Check sheet for the modelled part. Datum: model origin and axes. Units: mm. A direction names the side the tool comes from. Coordinates: 2 decimals unless noted, no trailing zeros. Loops run counter-clockwise (first coordinate to the right, second up) from the corner with the lowest first, then second, coordinate; pieces in that order, holes last. Notation, with made-up numbers: (-13, 32) - (22, 32) arc R35 ccw to (22, 65) - close; hole circle Ø1 at (83, 70.25). An arc over 180 degrees is marked (long way). Use a Markdown table: item, result. Add a question column.
1) Draft check along Y on faces 4 (the cylindrical face through (-3.78, -2.9, 21.41)), 5 (the flat face through (8, -8, 17.661)), 6 (the cylindrical face through (-0.448, 3.415, -33.518)). Enter one of: pulls with the +Y half, pulls with the -Y half, needs draft (parallel to the pull), parting line crosses it, or undercut.
2) Go/stop test with flat-tipped pins: P1, Ø3, axis at x = 0, y = 0, coming from the -Z side; P2, Ø3, axis at x = 1, y = -1, coming from the +Z side; P3, Ø8.5, axis at x = 0, y = 0, coming from the -Z side; P4, Ø8, axis at x = 22.5, y = -12, coming from the +Z side. Record where each tip stops, or that it passes through.
3) Tool access check on faces 1 (the cylindrical face through (25.034, 7.884, -11.992)), 2 (the flat face through (4, -4, 26.106)), 3 (the cylindrical face through (8.12, -3.37, 21.94)). Record the directions out of +Z, -Z, +X, -X, +Y, -Y that give a thin tool (end or side, any length) a straight path to the whole face; none if there is none.
4) Sectioned sample at A-A, the plane x = 24.5. Enter the section's corners in (y, z).
5) Sectioned sample at C-C, the plane z = -3. Enter the section's corners in (x, y), then the cut area to 3 significant figures.
6) Thickness scan on line 1 (Y direction, x = 0, z = 21); line 2 (Y direction, x = 0, z = -23); line 3 (Z direction, x = 28.5, y = 13.5). Record the ranges inside material, lowest first.
7) Sectioned sample at D-D, the plane z = -31.5. Enter the section's corners in (x, y) (1 decimal), then the cut area to 3 significant figures.
from build123d import *

# Parameters (mm, degrees)
F2_R     = 4.7625
F3_DEPTH = 9.525
F4_R     = 1.5875
F5_DEPTH = 22.225


with BuildPart() as f1:
    # F0 (on Front) → F1 (revolve)
    with BuildSketch(Plane.XZ):
        Polygon((8.793218, 26.10616), (0, 26.10616), (0, -37.513819), (3.444635, -37.513819), (3.444635, -29.631697), (7.104192, -29.631697), (7.104192, -21.186566), (16.393835, -21.186566), (16.393835, -15.274976), (26.246486, -15.274976), (26.246486, -8.800376), (33.565599, -8.800376), (33.565599, -4.296307), (36.099136, -4.296307), (36.099136, 17.661031), (8.793218, 17.661031), align=None)
    revolve(axis=Axis((0, 0, -5.703829), (0, 0, 1)))

    # F2 (on face) → F3 (cut)
    with BuildSketch(Plane.XY.offset(26.10616)):
        Circle(F2_R)
    extrude(amount=-F3_DEPTH, mode=Mode.SUBTRACT)

    # F4 (on face) → F5 (cut)
    with BuildSketch(Plane(origin=(0, 0, -37.513819), x_dir=(1, 0, 0), z_dir=(0, 0, -1))):
        Circle(F4_R)
    extrude(amount=-F5_DEPTH, mode=Mode.SUBTRACT)


solid = f1.part
Solved:
| question | item | result |
|---|---|---|
| 1 | face 4 | undercut |
| 1 | face 5 | needs draft |
| 1 | face 6 | parting line crosses it |
| 2 | P1 | stops at z = -15.29 |
| 2 | P2 | stops at z = 16.58 |
| 2 | P3 | stops at z = -37.51 |
| 2 | P4 | stops at z = 17.66 |
| 3 | face 1 | -Z |
| 3 | face 2 | +Z, +X, -X, +Y, -Y |
| 3 | face 3 | +Z |
| 4 | outline | (-26.51, -4.3) - (-22.94, -4.3) - (-22.94, -8.8) - (-9.41, -8.8) - (-9.41, -15.27) - (9.41, -15.27) - (9.41, -8.8) - (22.94, -8.8) - (22.94, -4.3) - (26.51, -4.3) - (26.51, 17.66) - (-26.51, 17.66) - close |
| 5 | outline | circle Ø72.2 at (0, 0) |
| 5 | area | 4,090 mm2 |
| 6 | line 1 | y = -8.79 to -4.76, 4.76 to 8.79 |
| 6 | line 2 | y = -7.1 to -1.59, 1.59 to 7.1 |
| 6 | line 3 | z = -8.8 to 17.66 |
| 7 | outline | circle Ø6.9 at (0, 0); hole circle Ø3.2 at (0, 0) |
| 7 | area | 29.4 mm2 |
